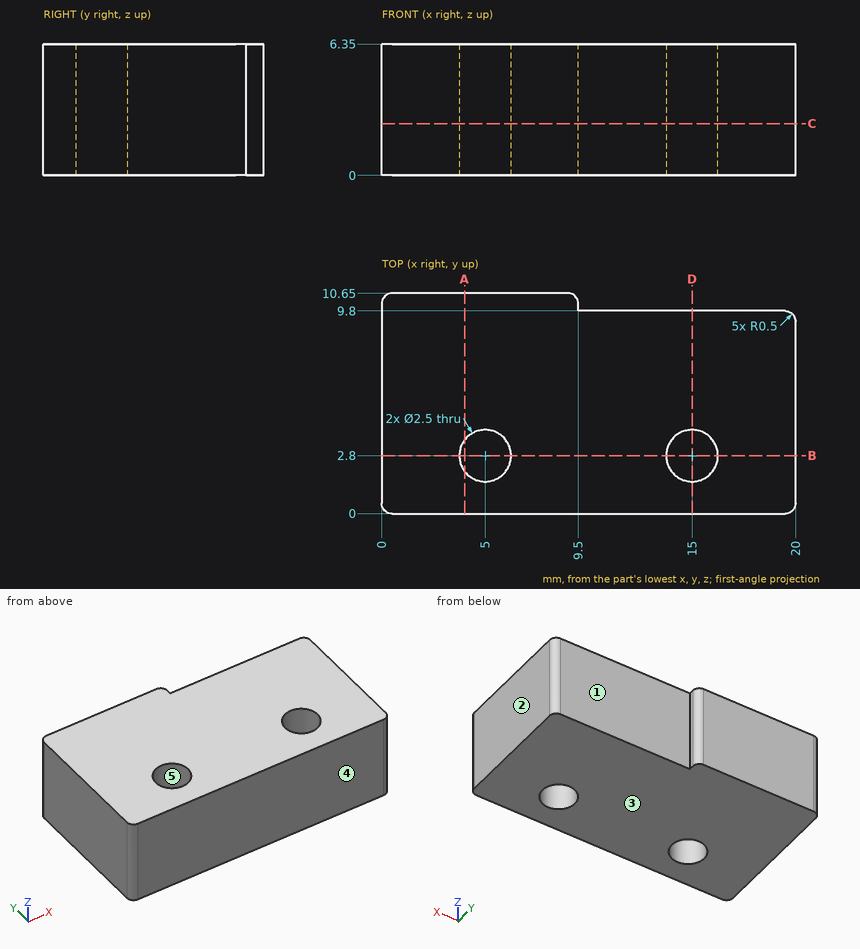
Answer from the drawing. Dimensions are ordinates in mm from the lowest x, y and z of the part. A direction names the side the tool comes from. Round coordinates to 2 decimals unless told otherwise and drop trailing zeros. Write each loop counter-clockwise with the first axis right and the second up, starting at its lowest first coordinate (ties: lowest second). Pieces come first, ordered by that corner, then holes. Notation, with made-up numbers: (76.25, 20.25) - (98.25, 20.25) arc R31 cw to (98.25, 55.25) - close; hole circle Ø8 at (-23, 6.5). An arc over 180 degrees is marked (long way). One line per item, written item: value.
Q1. Which of the six approach directions +Z, -Z, +X, -X, +Y, -Y give full straight-line access (tool end or side, diameter ignored) to the marked faces 1 and 2?
The answers:
face 1: +Z, -Z, +X, +Y
face 2: +Z, -Z, +X, +Y, -Y
Q2. Find section C-C (z = 2.5). Determine the outline of the cut face in (x, y), and give its area (3 significant figures).
The answers:
outline: (0, 0.5) arc R0.5 ccw to (0.5, 0) - (19.5, 0) arc R0.5 ccw to (20, 0.5) - (20, 9.3) arc R0.5 ccw to (19.5, 9.8) - (9.5, 9.8) - (9.5, 10.15) arc R0.5 ccw to (9, 10.65) - (0.5, 10.65) arc R0.5 ccw to (0, 10.15) - close; hole circle Ø2.5 at (5, 2.8); hole circle Ø2.5 at (15, 2.8)
area: 194 mm2
Q3. For a pull along Y with two mould halves and no side action, classify the marked faces 3, 4 and 5 as pulls with the +Y half, pulls with the -Y half, needs draft (parallel to the pull), parting line crosses it, or undercut.
The answers:
face 3: needs draft
face 4: pulls with the -Y half
face 5: undercut
Q4. Find section D-D (x = 15). Determine the outline of the cut face in (y, z).
The answers:
outline: (0, 0) - (1.55, 0) - (1.55, 6.35) - (0, 6.35) - close; (4.05, 0) - (9.8, 0) - (9.8, 6.35) - (4.05, 6.35) - close
Q5. Straight lines are drawn through the part: line 1 (Y direction, x = 5, z = 4.25); line 2 (Y direction, x = 15, z = 5); line 3 (X direction, y = 2, z = 2.75). For each, find the intervals that lie inside material, in ascending order. Write a range as from..to.
The answers:
line 1: y = 0..1.55, 4.05..10.65
line 2: y = 0..1.55, 4.05..9.8
line 3: x = 0..4.04, 5.96..14.04, 15.96..20
Q6. Find section B-B (y = 2.8). Determine the outline of the cut face in (x, z).
The answers:
outline: (0, 0) - (3.75, 0) - (3.75, 6.35) - (0, 6.35) - close; (6.25, 0) - (13.75, 0) - (13.75, 6.35) - (6.25, 6.35) - close; (16.25, 0) - (20, 0) - (20, 6.35) - (16.25, 6.35) - close
Q7. Find section A-A (x = 4). Determine the outline of the cut face in (y, z).
The answers:
outline: (0, 0) - (2.05, 0) - (2.05, 6.35) - (0, 6.35) - close; (3.55, 0) - (10.65, 0) - (10.65, 6.35) - (3.55, 6.35) - close
